from build123d import *

# Parameters (mm, degrees)
SKETCH1_W                                      = 107.95
SKETCH1_H                                      = 50.8
BOSS_EXTRUDE1_DEPTH                            = 9.525
SKETCH2_R                                      = 16.3195
CUT_EXTRUDE1_DEPTH                             = 19.05
SKETCH3_W                                      = 3.175
SKETCH3_H                                      = 25.4
CUT_EXTRUDE2_DEPTH                             = 19.05
CBORE_FOR_8_SOCKET_HEAD_CAP_SCREW1_D           = 4.4958
CBORE_FOR_8_SOCKET_HEAD_CAP_SCREW1_DEPTH       = 23.8125
CBORE_FOR_8_SOCKET_HEAD_CAP_SCREW1_CBORE_D     = 7.9375
CBORE_FOR_8_SOCKET_HEAD_CAP_SCREW1_CBORE_DEPTH = 4.1656
F_8_32_TAPPED_HOLE1_D                          = 3.4544
F_8_32_TAPPED_HOLE1_DEPTH                      = 25.4
F_8_32_TAPPED_HOLE1_TIP                        = 1.037806461
CUT_EXTRUDE3_DEPTH                             = 19.05


with BuildPart() as part:
    # Sketch1 → Boss-Extrude1 (new, symmetric)
    with BuildSketch(Plane(origin=(0, 0, 0), x_dir=(1, 0, 0), z_dir=(0, 1, 0))):
        Rectangle(SKETCH1_W, SKETCH1_H)
    extrude(amount=BOSS_EXTRUDE1_DEPTH, both=True)

    # Sketch2 → Cut-Extrude1 (cut)
    with BuildSketch(Plane(origin=(0, 9.525, 0), x_dir=(1, 0, 0), z_dir=(0, 1, 0))):
        with Locations(Location((-28.575, 0, 0), (0, 0, 270))):
            Circle(SKETCH2_R)
    extrude(amount=-CUT_EXTRUDE1_DEPTH, mode=Mode.SUBTRACT)

    # Sketch3 → Cut-Extrude2 (cut)
    with BuildSketch(Plane(origin=(0, 9.525, 0), x_dir=(1, 0, 0), z_dir=(0, 1, 0))):
        with Locations((-28.575, -12.7)):
            Rectangle(SKETCH3_W, SKETCH3_H)
    extrude(amount=-CUT_EXTRUDE2_DEPTH, mode=Mode.SUBTRACT)

    # CBORE for #8 Socket Head Cap Screw1
    with Locations(Plane.ZY.offset(53.975)):
        with Locations((20.6375, 0)):
            CounterBoreHole(CBORE_FOR_8_SOCKET_HEAD_CAP_SCREW1_D / 2, CBORE_FOR_8_SOCKET_HEAD_CAP_SCREW1_CBORE_D / 2, CBORE_FOR_8_SOCKET_HEAD_CAP_SCREW1_CBORE_DEPTH, depth=CBORE_FOR_8_SOCKET_HEAD_CAP_SCREW1_DEPTH)

    # #8-32 Tapped Hole1
    with Locations(Plane.ZY.offset(26.9875)):
        with Locations((20.6375, 0)):
            Hole(F_8_32_TAPPED_HOLE1_D / 2, depth=F_8_32_TAPPED_HOLE1_DEPTH)
            with Locations((0, 0, -(F_8_32_TAPPED_HOLE1_DEPTH + F_8_32_TAPPED_HOLE1_TIP / 2))):  # 118° drill point
                Cone(0, F_8_32_TAPPED_HOLE1_D / 2, F_8_32_TAPPED_HOLE1_TIP, mode=Mode.SUBTRACT)

    # Sketch12 → Cut-Extrude3 (cut)
    with BuildSketch(Plane(origin=(0, 9.525, 0), x_dir=(1, 0, 0), z_dir=(0, 1, 0))):
        with BuildLine():
            Line((6.35, 3.2639), (44.45, 3.2639))
            ThreePointArc((44.45, 3.2639), (47.7139, 0), (44.45, -3.2639))
            Line((44.45, -3.2639), (6.35, -3.2639))
            ThreePointArc((6.35, -3.2639), (3.0861, 0), (6.35, 3.2639))
        make_face()
    extrude(amount=-CUT_EXTRUDE3_DEPTH, mode=Mode.SUBTRACT)


solid = part.part
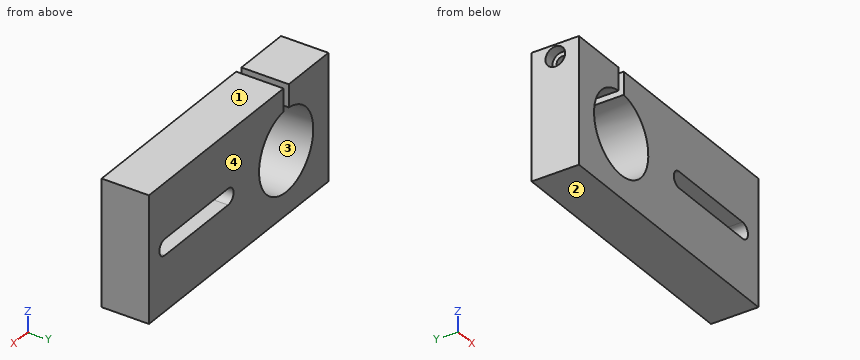
Read the model definition and answer for the solid it produces. Units are mm, in the model's axes. Face numbers are marked on the shaded views. Round coordinates to 2 decimals unless told otherwise and drop trailing zeros. Write each loop counter-clockwise with the first axis right and the second up, starting at its lowest first coordinate (ties: lowest second). Pieces come first, ordered by that corner, then holes.
1. Determine the mould class of the marked faces 1, 2, 3 and 4 for opening direction Z: pulls with the +Z half, pulls with the -Z half, needs draft (parallel to the pull), parting line crosses it, or undercut.
2. Given pin 1 Ø2.5 at (y, z) = (-1, 20) entering from -X; pin 2 Ø4 at (y, z) = (0, 20.64) entering from -X, each flat-ended and moving along its own axis, determine where each tip first touches the part or whether it passes through.
3. The part is cut by section B-B, the plane x = 31.5. Determine the outline of the cut face in (y, z) (3 decimals).
4. The part is cut by section A-A, the plane z = 0. Determine the outline of the cut face in (x, y) (1 decimal), then the cut area to 3 significant figures.
5. Straight lines are drawn through the part: L1, parallel to X at y = -1.5, z = 0 (1 decimal); L2, parallel to Z at x = 28.5, y = 8.25; L3, parallel to X at y = -4.75, z = 1 (3 decimals). For each, find the intervals that lie inside material, in ascending order.
6. The part is cut by section D-D, the plane x = -36.5. Determine the outline of the cut face in (y, z) (1 decimal).
Values:
1. face 1: pulls with the +Z half
1. face 2: pulls with the -Z half
1. face 3: undercut
1. face 4: needs draft
2. pin 1: stops at x = -49.81
2. pin 2: stops at x = -26.99
3. outline: (-9.525, -25.4) - (9.525, -25.4) - (9.525, -3.264) - (-9.525, -3.264) - close; (-9.525, 3.264) - (9.525, 3.264) - (9.525, 25.4) - (-9.525, 25.4) - close
4. outline: (-54, -9.5) - (-44.9, -9.5) - (-44.9, 9.5) - (-54, 9.5) - close; (-12.3, -9.5) - (3.1, -9.5) - (3.1, 9.5) - (-12.3, 9.5) - close; (47.7, -9.5) - (54, -9.5) - (54, 9.5) - (47.7, 9.5) - close
4. area: 585 mm2
5. L1: x = -54 to -44.9, -12.3 to 3.1, 47.7 to 54
5. L2: z = -25.4 to -3.26, 3.26 to 25.4
5. L3: x = -53.975 to -44.864, -12.286 to 3.243, 47.557 to 53.975
6. outline: (-9.5, -25.4) - (9.5, -25.4) - (9.5, -14.3) - (-9.5, -14.3) - close; (-9.5, 14.3) - (9.5, 14.3) - (9.5, 25.4) - (-9.5, 25.4) - close; hole circle Ø4.5 at (0, 20.6)
